Print and shaded views of the part. All mm, measured from the part's lowest x, y and z. Round coordinates to 2 decimals unless told otherwise and drop trailing zeros. Write each loop counter-clockwise with the first axis right and the second up, starting at its lowest first coordinate (ties: lowest second). Pieces come first, ordered by that corner, then holes. Notation, with made-up numbers: (76.25, 55) - (119.25, 55) arc R22 cw to (119.25, 84) - close; hole circle Ø4 at (86, 42.25). An arc over 180 degrees is marked (long way). Answer as a JSON object with one key per item and string values. Group by question number.
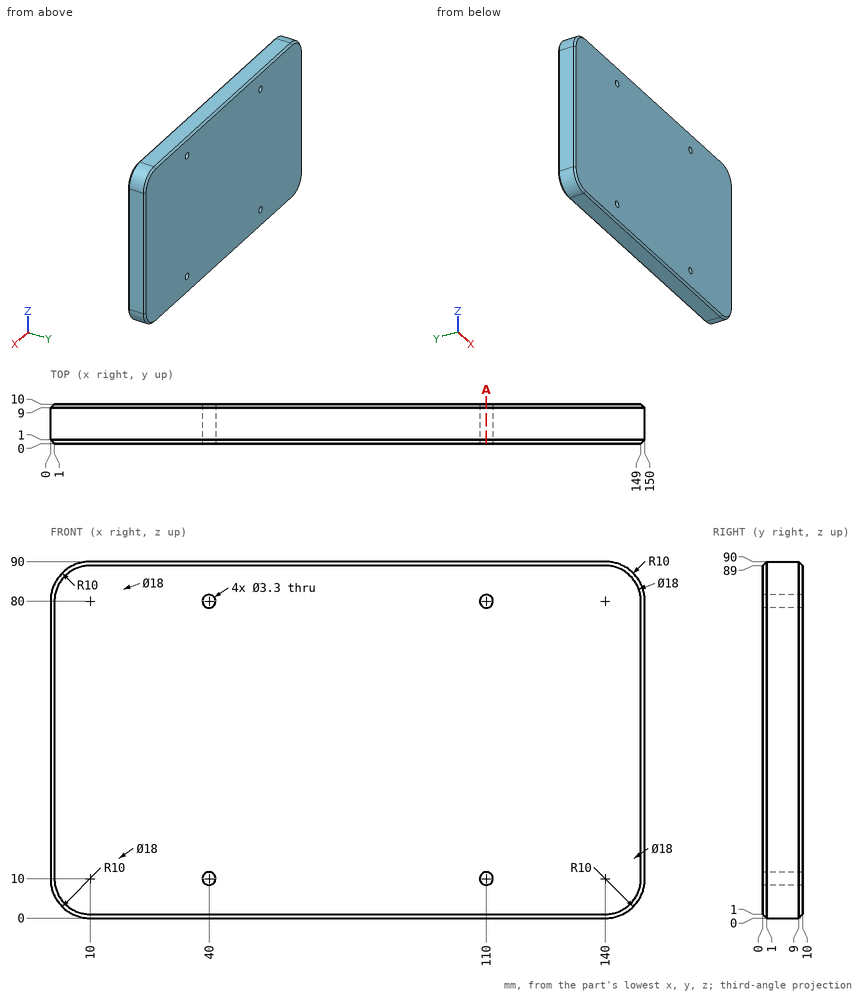
(1) Flat gauge pin, fed straight in: pin 1 (3 mm diameter, centred on x = 110, z = 10, fed in from +Y). Where does the tip first touch, or does it go through?
(2) Slice it at A-A (x = 110). Write the cut outline in (y, z).
(3) Drill centre lines: line 1 (X direction, y = 5, z = 80); line 2 (Z direction, x = 110, y = 7.25); line 3 (Z direction, x = 79.5, y = 9.75). Where is each one in solid material? Low to high. Write a range as from..to.
Answer:
{
 "1": {"pin 1": "through"},
 "2": {"outline": "(0, 1) - (1, 0) - (9, 0) - (10, 1) - (10, 8.35) - (0, 8.35) - close; (0, 11.65) - (10, 11.65) - (10, 78.35) - (0, 78.35) - close; (0, 81.65) - (10, 81.65) - (10, 89) - (9, 90) - (1, 90) - (0, 89) - close"},
 "3": {"line 1": "0..38.35, 41.65..108.35, 111.65..150", "line 2": "0..8.35, 11.65..78.35, 81.65..90", "line 3": "0.75..89.25"}
}
